Build history of the part. All positions in model axes, mm. A direction names the side the tool comes from. Round coordinates to 2 decimals unless told otherwise and drop trailing zeros. Order: outer loops, then holes, each group sorted by start corner. A loop starts at its lowest first (then second) coordinate and runs counter-clockwise, first axis right, second up. Notation, with made-up numbers: M 75.5,26 L 131.5,26 A30 ccw 131.5,64 Z; hole C 5,85 d9. An arc over 180 degrees is marked long. Use CSV: the item, a comma, the result in double quotes.
Autodesk Inventor part; units mm, degrees
ref_plane "YZ Plane" through (0, 0, 0) normal (1, 0, 0) x (0, 1, 0)
ref_plane "XZ Plane" through (0, 0, 0) normal (0, 1, 0) x (-1, 0, 0)
ref_plane "XY Plane" through (0, 0, 0) normal (0, 0, 1) x (1, 0, 0)
sketch "Sketch1" plane through (0, 0, 0) normal (0, 1, 0) x (-1, 0, 0)
  circle A0 centre (0, 0) radius 10.25
  dimension "d0" = 20.5
extrude "Extrusion1" add sketch "Sketch1" along normal blind 7.05
sketch "Sketch2" plane through (0, 7.05, 0) normal (0, 1, 0) x (1, 0, 0)
  circle A0 centre (0, 0) radius 12.475
  dimension "d3" = 24.95
extrude "Extrusion2" add sketch "Sketch2" along normal blind 4
sketch "Sketch3" plane through (0, 11.05, 0) normal (0, 1, 0) x (1, 0, 0)
  circle A0 centre (0, 0) radius 12.475
  line L0 (-12.5, -12.5) -> (12.5, -12.5)
  line L1 (12.5, -12.5) -> (12.5, 12.5)
  line L2 (12.5, 12.5) -> (-12.5, 12.5)
  line L3 (-12.5, 12.5) -> (-12.5, -12.5)
  point P0 (-12.5, 0)
  point P1 (0, -12.5)
  dimension "d6" = 25
  dimension "d7" = 25
extrude "Extrusion3" add sketch "Sketch3" along normal blind 6.1 contours A0 | L3 L2 L1 L0
sketch "Sketch4" plane through (12.5, 11.05, 12.5) normal (1, 0, 0) x (0, 0, -1)
  line L0 (0, 0) -> (25, 0)
  line L1 (25, 0) -> (25, 6.1)
  line L2 (0, 6.1) -> (25, 6.1)
  line L3 (0, 0) -> (0, 6.1)
  line L4 (24.975, 0) -> (0.025, 0)
  line L5 (6.5, 0) -> (18.5, 0)
  line L6 (18.5, 0) -> (18.5, 3)
  line L7 (18.5, 3) -> (6.5, 3)
  line L8 (6.5, 3) -> (6.5, 0)
  point P0 (12.5, -11.05)
  point P1 (12.5, 3)
  point P2 (12.5, 0)
  point P3 (12.5, 0)
  dimension "d10" = 12
  dimension "d11" = 3
hole "Hole1" at (12.5, 14.05, 6) at (12.5, 14.05, -6) direction (-1, 0, 0) diameter 1.567 end through all
sketch "Sketch5" plane through (0, 0, 0) normal (0, -1, 0) x (1, 0, 0)
  circle A0 centre (0, 0) radius 3.5
  dimension "d19" = 7
extrude "Extrusion4" cut sketch "Sketch5" against normal blind 2.5
sketch "Sketch6" plane through (0, 0, 0) normal (0, -1, 0) x (1, 0, 0)
  circle A0 centre (0, 0) radius 7
  line L0 (0, 7) -> (-7, 0)
  line L1 (-7, 0) -> (0, -7)
  line L2 (0, -7) -> (7, 0)
  line L3 (7, 0) -> (0, 7)
  dimension "d22" = 14
hole "Hole2" at (0, 0, 7) at (-7, 0, 0) at (0, 0, -7) at (7, 0, 0) direction (0, 1, 0) diameter 3.1 end through all
sketch "Sketch7" plane through (0, 17.15, 0) normal (0, 1, 0) x (1, 0, 0)
  circle A0 centre (0, 7) radius 1.55
  circle A1 centre (0, -7) radius 1.55
  circle A2 centre (-7, 0) radius 1.55
  circle A3 centre (7, 0) radius 1.55
  line L0 (-12.5, -12.5) -> (12.5, -12.5)
  line L1 (12.5, -12.5) -> (12.5, 12.5)
  line L2 (12.5, 12.5) -> (-12.5, 12.5)
  line L3 (-12.5, 12.5) -> (-12.5, -12.5)
  point P0 (0, 0)
hole "Hole3" at (0, 17.15, 7) at (7, 17.15, 0) at (0, 17.15, -7) at (-7, 17.15, 0) direction (0, -1, 0) diameter 5.7 depth 3.2 tip angle 100
equation "\"d7\" = d6"
properties part number "c_axisrot"
(1) Cut at B-B, the plane x = 0. Count the separate pieces of the cut face and the enclosed holes in it, and give its area (3 significant figures).
Answer block:
separate pieces,"3"
enclosed holes,"0"
area,"254 mm²"
(2) Cut at A-A, the plane y = 12. Give the cut face in (x, z).
Answer block:
outline,"M -12.5,-12.5 L 12.5,-12.5 L 12.5,12.5 L -12.5,12.5 Z; hole C -7,0 d3.1; hole C 0,-7 d3.1; hole C 0,7 d3.1; hole C 7,0 d3.1"
(3) Wall check: line 1 (Z direction, x = 0, y = 15); line 2 (Z direction, x = 0, y = 6.75); line 3 (Z direction, x = -7.25, y = 14.05). Give the ranges that are in metal, low to high. Write a range as from..to.
Answer block:
line 1,"z = -12.5..-9.85, -4.15..4.15, 9.85..12.5"
line 2,"z = -10.25..-8.55, -5.45..5.45, 8.55..10.25"
line 3,"z = -12.5..-6.78, -5.22..-2.84, 2.84..5.22, 6.78..12.5"
(4) Cut at C-C, the plane x = -7. Give the cut face in (y, z).
Answer block:
outline,"M 0,-7.49 L 7.05,-7.49 L 7.05,-10.33 L 11.05,-10.33 L 11.05,-12.5 L 17.15,-12.5 L 17.15,-2.85 L 13.95,-2.85 L 12.86,-1.55 L 0,-1.55 Z; M 0,1.55 L 12.86,1.55 L 13.95,2.85 L 17.15,2.85 L 17.15,12.5 L 11.05,12.5 L 11.05,10.33 L 7.05,10.33 L 7.05,7.49 L 0,7.49 Z; hole C 14.05,-6 d1.57; hole C 14.05,6 d1.57"
(5) Two-plate mould, pull along Y, no slides. Class faces 1 (the face through (7, 13.273, -5.898)), 2 (the face through (4.174, 15.528, -0.371)), 3 (the face through (0.078, 13.049, -8.774)): released by +Y, released by -Y, zero draft, split by the parting line, or undercut.
Answer block:
face 1,"undercut"
face 2,"zero draft"
face 3,"released by +Y"
(6) Tool access for faces 4 (the face through (-7.152, 13.273, -5.898)), 5 (the face through (1.092, 15.528, 9.633)), 6 (the face through (0, 2.5, 0)): list every direction of +Z, -Z, +X, -X, +Y, -Y with a clear straight run to the whole face (end or side of a thin tool).
Answer block:
face 4,"+X, -X"
face 5,"+Y"
face 6,"-Y"
(7) Drop flat-ended pins along their axis: pin 1 (9 mm diameter, centred on x = -7, z = 0, fed in from +Y); pin 2 (3.5 mm diameter, centred on x = -7, z = 0, fed in from +Y); pin 3 (2 mm diameter, centred on x = 1, y = 3, fed in from -Z); pin 4 (2 mm diameter, centred on x = 1, z = -0.5, fed in from -Y). Give the stop position or say it passes through.
Answer block:
pin 1,"stops at y = 17.15"
pin 2,"stops at y = 13.03"
pin 3,"stops at z = -10.25"
pin 4,"stops at y = 2.5"
